Design review of the part built by this model. Coordinates are the model's own, in mm. A direction names the side the tool comes from. Round coordinates to 2 decimals unless told otherwise and drop trailing zeros. Loops run counter-clockwise (first coordinate to the right, second up) from the corner with the lowest first, then second, coordinate; pieces in that order, holes last. Notation, with made-up numbers: (-2.75, -28.5) - (9.25, -28.5) arc R3 ccw to (9.25, -24.5) - close; hole circle Ø9 at (14.25, 30.25). An arc over 180 degrees is marked (long way). Use one line per item in the form item = value. Start each with the question number.
(1) We need section A-A, the plane z = 0. Write out the cut boundary in (x, y).
(2) For pin 1 (8 mm diameter, centred on x = 5.5, y = -6.5, fed in from -Z); pin 2 (2 mm diameter, centred on y = -2, z = 13, fed in from +X); pin 3 (3 mm diameter, centred on x = 0.5, z = -13.5, fed in from +Y); pin 4 (2 mm diameter, centred on x = -4, y = -17, fed in from -Z), all flat-tipped, find the tip position at first contact; note any pin that passes through.
(3) Wall thickness on probe 1 along Y at (x, z) = (-11.8, 13); probe 2 along Z at (x, y) = (0, -4.25): over which ranges is each line inside the solid? List them lowest first. Write a range as [from, to].
(4) The part is to be moulded in two halves that separate along X. For faces 1 (the flat face through (-4.1, -19, 0)), 2 (the cylindrical face through (-12.19, -2.67, 13.87)), 3 (the flat face through (-4.3, -18.6, -0.1)), say which applies: released by +X, released by -X, zero draft, split by the parting line, or undercut.
(5) Machinability: for faces 4 (the cylindrical face through (16.116, -14.173, -2.05)), 5 (the cylindrical face through (17.23, -7, 0.15)), 6 (the flat face through (4.1, -19, 0)), 7 (the flat face through (4.5, -20, -0.3)), which of the approach directions +Z, -Z, +X, -X, +Y, -Y give a long, thin tool a straight path to every point of the face, cutting with its end or side? Answer none if there is none.
(6) We need section D-D, the plane y = -15. Write out the cut boundary in (x, z).
(7) We need section B-B, the plane x = 0.5. Write out the cut boundary in (y, z).
(8) We need section C-C, the plane y = -2. Write out the cut boundary in (x, z), then the cut area to 3 significant figures.
from build123d import *

# Parameters (mm, degrees)
SKETCH3_R                            = 19
MAIN_BODY_DEPTH                      = 20
CUT_START                            = -7.7
SKETCH5_R                            = 17
CUT_FOR_HEADERS_DEPTH                = 26.796268449
CUT_FOR_ADNS_WIRES_REACH             = 35.496
CUT_FOR_ADNS_WIRES_END_RADIUS        = 19
SKETCH7_R                            = 7
SKETCH8_R                            = 15.75
CUT_FOR_PCB_DEPTH                    = 3.8
SKETCH9_R                            = 1.25
CUT_FOR_SCREW_HOLES_DEPTH            = 5
SKETCH10_W                           = 18.9
SKETCH10_H                           = 21.2
CUT_FOR_LENS_DEPTH                   = 2.5
CUT_FOR_PUPIL_REACH                  = 34.68
SKETCH11_W                           = 8.2
SKETCH11_H                           = 10.2
CUTS_FOR_BODY_SCREW_HOLES_DEPTH      = 34.496268622
CUTS_FOR_BODY_SCREW_HOLES_DEPTH_BACK = 34.496268622
SKETCH13_R                           = 1.1


with BuildPart() as part:
    # Sketch3 → Main Body (new body)
    with BuildSketch(Plane(origin=(0, 0, 0), x_dir=(1, 0, 0), z_dir=(0, 1, 0))):
        with Locations(Location((0, 0, 0), (0, 0, 270))):
            Circle(SKETCH3_R)
    extrude(amount=-MAIN_BODY_DEPTH)

    # Sketch5 → Cut for Headers (cut, through all)
    with BuildSketch(Plane.XZ.offset(20).offset(CUT_START)):
        with Locations(Location((0, 0, 0), (0, 0, 270))):
            Circle(SKETCH5_R)
    extrude(amount=-CUT_FOR_HEADERS_DEPTH, mode=Mode.SUBTRACT)

    # Cut for ADNS Wires: up to this cylinder (the profile starts inside it)
    cut_for_adns_wires_end = Plane(origin=(0, 0, 0), z_dir=(0, 1, 0)) * Cylinder(CUT_FOR_ADNS_WIRES_END_RADIUS, 109.992, mode=Mode.PRIVATE)
    # Sketch7 → Cut for ADNS Wires (cut, up to the surface)
    with BuildSketch(Plane(origin=(0, 0, 0), x_dir=(0, 0, -1), z_dir=(1, 0, 0)), mode=Mode.PRIVATE) as cut_for_adns_wires_sk1:
        Circle(SKETCH7_R)
    cut_for_adns_wires_tool1 = extrude(cut_for_adns_wires_sk1.sketch, amount=CUT_FOR_ADNS_WIRES_REACH, mode=Mode.PRIVATE) & cut_for_adns_wires_end
    add(cut_for_adns_wires_tool1.solids().sort_by_distance((0, 0, 0))[0], mode=Mode.SUBTRACT)

    # Sketch8 → Cut for PCB (cut)
    with BuildSketch(Plane(origin=(0, -12.3, 0), x_dir=(1, 0, 0), z_dir=(0, 1, 0))):
        with Locations(Location((0.5, 0, 0), (0, 0, 270))):
            Circle(SKETCH8_R)
    extrude(amount=-CUT_FOR_PCB_DEPTH, mode=Mode.SUBTRACT)

    # Sketch9 → Cut for Screw Holes (cut)
    with BuildSketch(Plane(origin=(0, -16.1, 0), x_dir=(1, 0, 0), z_dir=(0, 1, 0))):
        with Locations(Location((0.5, 13.5, 0), (0, 0, 270))):
            Circle(SKETCH9_R)
        with Locations(Location((0.5, -13.5, 0), (0, 0, 270))):
            Circle(SKETCH9_R)
    extrude(amount=-CUT_FOR_SCREW_HOLES_DEPTH, mode=Mode.SUBTRACT)

    # Sketch10 → Cut for Lens (cut)
    with BuildSketch(Plane(origin=(0, -16.1, 0), x_dir=(1, 0, 0), z_dir=(0, 1, 0))):
        Rectangle(SKETCH10_W, SKETCH10_H)
    extrude(amount=-CUT_FOR_LENS_DEPTH, mode=Mode.SUBTRACT)

    # Sketch11 → Cut for Pupil (cut, up to next)
    with BuildSketch(Plane(origin=(0, -18.6, 0), x_dir=(1, 0, 0), z_dir=(0, 1, 0)), mode=Mode.PRIVATE) as cut_for_pupil_sk1:
        Rectangle(SKETCH11_W, SKETCH11_H)
    cut_for_pupil_tool1 = extrude(cut_for_pupil_sk1.sketch, amount=-CUT_FOR_PUPIL_REACH, mode=Mode.PRIVATE) & part.part
    add(cut_for_pupil_tool1.solids().sort_by_distance((0, -18.6, 0))[0], mode=Mode.SUBTRACT)

    # Sketch13 → Cuts for Body Screw Holes (cut, two sides: drawn at the far end of the back side and taken through both)
    with BuildSketch(Plane(origin=(0, 0, 0), x_dir=(0, 0, -1), z_dir=(1, 0, 0)).offset(-CUTS_FOR_BODY_SCREW_HOLES_DEPTH_BACK)):
        with Locations((13, -2)):
            Circle(SKETCH13_R)
        with Locations((-13, -2)):
            Circle(SKETCH13_R)
    extrude(amount=CUTS_FOR_BODY_SCREW_HOLES_DEPTH + CUTS_FOR_BODY_SCREW_HOLES_DEPTH_BACK, mode=Mode.SUBTRACT)


solid = part.part
Data:
q1.outline = (-19, -20) - (-4.1, -20) - (-4.1, -18.6) - (-9.45, -18.6) - (-9.45, -16.1) - (-15.25, -16.1) - (-15.25, -12.3) - (-17, -12.3) - (-17, 0) - (-19, 0) - close; (4.1, -20) - (19, -20) - (19, -7) - (17, -7) - (17, -12.3) - (16.25, -12.3) - (16.25, -16.1) - (9.45, -16.1) - (9.45, -18.6) - (4.1, -18.6) - close
q2.pin_1 = -18.94
q2.pin_2 = through
q2.pin_3 = -16.1
q2.pin_4 = -18.76
q3.probe_1 = [-20, -3.1], [-0.9, 0]
q3.probe_2 = [-19, -17], [17, 19]
q4.face_1 = undercut
q4.face_2 = zero draft
q4.face_3 = undercut
q5.face_4 = +Y
q5.face_5 = +X, +Y
q5.face_6 = +Y, -Y
q5.face_7 = +Z, -Z, +X, -X, -Y
q6.outline = circle Ø38 at (0, 0); hole circle Ø31.5 at (0.5, 0)
q7.outline = (-20, -18.99) - (0, -18.99) - (0, -16.99) - (-12.3, -16.99) - (-12.3, -15.75) - (-16.1, -15.75) - (-16.1, -14.75) - (-20, -14.75) - close; (-20, -12.25) - (-16.1, -12.25) - (-16.1, -10.6) - (-18.6, -10.6) - (-18.6, -5.1) - (-20, -5.1) - close; (-20, 5.1) - (-18.6, 5.1) - (-18.6, 10.6) - (-16.1, 10.6) - (-16.1, 12.25) - (-20, 12.25) - close; (-20, 14.75) - (-16.1, 14.75) - (-16.1, 15.75) - (-12.3, 15.75) - (-12.3, 16.99) - (0, 16.99) - (0, 18.99) - (-20, 18.99) - close
q8.outline = (-14.81, -11.9) - (-12.14, -11.9) arc R17 cw to (-12.14, 11.9) - (-14.81, 11.9) arc R19 ccw to start; (-12.74, -14.1) arc R19 ccw to (12.74, -14.1) - (9.5, -14.1) arc R17 cw to (-9.5, -14.1) - close; (-12.74, 14.1) - (-9.5, 14.1) arc R17 cw to (9.5, 14.1) - (12.74, 14.1) arc R19 ccw to start; (12.14, -11.9) - (14.81, -11.9) arc R19 ccw to (17.78, -6.71) - (15.62, -6.71) arc R17 cw to start; (12.14, 11.9) arc R17 cw to (15.62, 6.71) - (17.78, 6.71) arc R19 ccw to (14.81, 11.9) - close
q8.area = 173 mm^2
